The model under review builds one solid part; all positions refer to its coordinate system, in mm. Face numbers are marked on the shaded views. A direction names the side the tool comes from. Coordinates: 2 decimals unless noted, no trailing zeros. Order: outer loops, then holes, each group sorted by start corner. A loop starts at its lowest first (then second) coordinate and runs counter-clockwise, first axis right, second up.
```python
from build123d import *

# Parameters (mm, degrees)
BOSS_EXTRUDE1_DEPTH                      = 42
CBORE_FOR_M64_HEX_HEAD_BOLT1_D           = 70
CBORE_FOR_M64_HEX_HEAD_BOLT1_CBORE_D     = 110
CBORE_FOR_M64_HEX_HEAD_BOLT1_CBORE_DEPTH = 7.5
F_16_5_16_5_DIAMETER_HOLE1_REACH         = 188.325
F_16_5_16_5_DIAMETER_HOLE1_BORE_R        = 8.25
M6_CLEARANCE_HOLE1_D                     = 6.647
M6_CLEARANCE_HOLE1_DEPTH                 = 22.2
M6_CLEARANCE_HOLE1_TIP                   = 1.996960267
CHAMFER1_SIZE                            = 0.5
CHAMFER2_SIZE                            = 1.1765
CHAMFER3_SIZE                            = 0.25


with BuildPart() as part:
    # Sketch1 → Boss-Extrude1 (new body)
    with BuildSketch(Plane(origin=(0, 0, -111.250000238), x_dir=(-1, 0, 0), z_dir=(0, 0, -1))):
        with BuildLine():
            Line((-55.395346272, -72.559925727), (37.878444259, -72.559925727))
            ThreePointArc((37.878444259, -72.559925727), (47.810091488, -64.128468222), (56.241548993, -54.196820993))
            Line((56.241548993, -54.196820993), (56.241548993, 39.076969538))
            ThreePointArc((56.241548993, 39.076969538), (47.810091488, 49.008616768), (37.878444259, 57.440074273))
            Line((37.878444259, 57.440074273), (-55.395346272, 57.440074273))
            ThreePointArc((-55.395346272, 57.440074273), (-65.326993501, 49.008616768), (-73.758451007, 39.076969538))
            Line((-73.758451007, 39.076969538), (-73.758451007, -54.196820993))
            ThreePointArc((-73.758451007, -54.196820993), (-65.326993501, -64.128468222), (-55.395346272, -72.559925727))
        make_face()
    extrude(amount=-BOSS_EXTRUDE1_DEPTH)

    # CBORE for M64 Hex Head Bolt1 (through all)
    with Locations(Plane(origin=(0, 0, -111.250000238), x_dir=(-1, 0, 0), z_dir=(0, 0, -1))):
        with Locations((-8.758451007, -7.559925727)):
            CounterBoreHole(CBORE_FOR_M64_HEX_HEAD_BOLT1_D / 2, CBORE_FOR_M64_HEX_HEAD_BOLT1_CBORE_D / 2, CBORE_FOR_M64_HEX_HEAD_BOLT1_CBORE_DEPTH)

    # Ø16.5 (16.5) Diameter Hole1 bore → Ø16.5 (16.5) Diameter Hole1 (cut, up to next)
    with BuildSketch(Plane(origin=(0, 57.440074273, 0), x_dir=(1, 0, 0), z_dir=(0, 1, 0)), mode=Mode.PRIVATE) as f_16_5_16_5_diameter_hole1_sk1:
        with Locations((-10.241548993, 83.250000238)):
            Circle(F_16_5_16_5_DIAMETER_HOLE1_BORE_R)
    f_16_5_16_5_diameter_hole1_tool1 = extrude(f_16_5_16_5_diameter_hole1_sk1.sketch, amount=-F_16_5_16_5_DIAMETER_HOLE1_REACH, mode=Mode.PRIVATE) & part.part
    add(f_16_5_16_5_diameter_hole1_tool1.solids().sort_by_distance((-10.241549, 57.440074, -83.25))[0], mode=Mode.SUBTRACT)

    # M6 Clearance Hole1
    with Locations(Plane(origin=(0, 0, -111.250000238), x_dir=(-1, 0, 0), z_dir=(0, 0, -1))):
        with Locations((42.506790629, -58.825167363), (-60.023692643, -58.825167363), (-60.023692643, 43.705315909), (42.506790629, 43.705315909)):
            Hole(M6_CLEARANCE_HOLE1_D / 2, depth=M6_CLEARANCE_HOLE1_DEPTH)
            with Locations((0, 0, -(M6_CLEARANCE_HOLE1_DEPTH + M6_CLEARANCE_HOLE1_TIP / 2))):  # 118° drill point
                Cone(0, M6_CLEARANCE_HOLE1_D / 2, M6_CLEARANCE_HOLE1_TIP, mode=Mode.SUBTRACT)

    # Chamfer1
    chamfer1_edges = [part.edges().sort_by_distance(p)[0] for p in [
        (-56.241548993, -7.559925727, -111.250000238),
        (-47.810091488, -64.128468222, -111.250000238),
        (8.758451007, -72.559925727, -111.250000238),
        (65.326993501, -64.128468222, -111.250000238),
        (63.758451007, -7.559925727, -111.250000238),
        (-26.241548993, -7.559925727, -103.750000238),
        (73.758451007, -7.559925727, -111.250000238),
        (65.326993501, 49.008616768, -111.250000238),
        (8.758451007, 57.440074273, -111.250000238),
        (-47.810091488, 49.008616768, -111.250000238),
    ]]
    chamfer(chamfer1_edges, length=CHAMFER1_SIZE)

    # Chamfer2
    chamfer2_edges = [part.edges().sort_by_distance(p)[0] for p in [
        (-45.830290629, 43.705315909, -111.250000238),
        (56.700192643, 43.705315909, -111.250000238),
        (56.700192643, -58.825167363, -111.250000238),
        (-45.830290629, -58.825167363, -111.250000238),
    ]]
    chamfer(chamfer2_edges, length=CHAMFER2_SIZE)

    # Chamfer3
    chamfer3_edges = [part.edges().sort_by_distance(p)[0] for p in [
        (-18.491548993, 57.440074273, -83.250000238),
    ]]
    chamfer(chamfer3_edges, length=CHAMFER3_SIZE)


solid = part.part
```
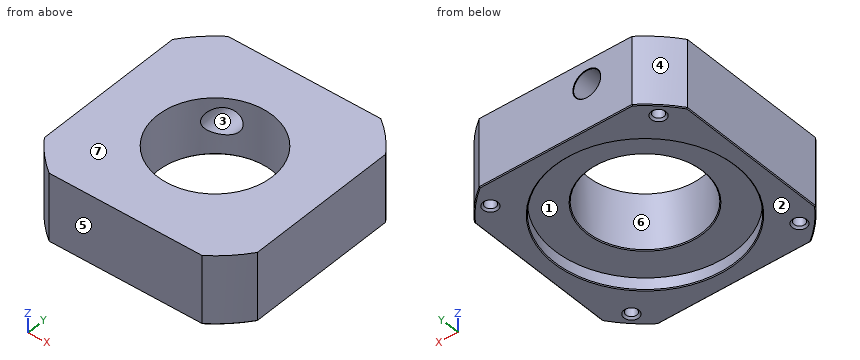
(1) Machinability: for the marked faces 1, 2 and 3, which of the approach directions +Z, -Z, +X, -X, +Y, -Y give a long, thin tool a straight path to every point of the face, cutting with its end or side? Answer none if there is none.
A:
face 1: -Z
face 2: -Z, +X, -X, +Y, -Y
face 3: +Y
(2) We need section C-C, the plane x = -15. Count the separate pieces of the cut face and the enclosed holes in it, and give its area (3 significant figures).
A:
separate pieces: 3
enclosed holes: 0
area: 2,410 mm2
(3) We need section B-B, the plane z = -83.25. Write out the cut boundary in (x, y), and give its area (3 significant figures).
A:
outline: (-56.24, -54.2) arc R80 ccw to (-37.88, -72.56) - (55.4, -72.56) arc R80 ccw to (73.76, -54.2) - (73.76, 39.08) arc R80 ccw to (55.4, 57.44) - (-1.74, 57.44) - (-1.99, 57.19) - (-1.99, 25.75) arc R35 cw (long way) to (-18.49, 14.4) - (-18.49, 57.19) - (-18.74, 57.44) - (-37.88, 57.44) arc R80 ccw to (-56.24, 39.08) - close
area: 11,900 mm2
(4) We need section A-A, the plane z = -73. Write out the cut boundary in (x, y).
A:
outline: (-56.24, -54.2) arc R80 ccw to (-37.88, -72.56) - (55.4, -72.56) arc R80 ccw to (73.76, -54.2) - (73.76, 39.08) arc R80 ccw to (55.4, 57.44) - (-37.88, 57.44) arc R80 ccw to (-56.24, 39.08) - close; hole circle Ø70 at (8.76, -7.56)
(5) For pin 1 Ø6 at (x, y) = (60.02, 43.71) entering from -Z; pin 2 Ø1 at (x, z) = (59.5, -92) entering from -Y; pin 3 Ø15 at (x, z) = (-10.24, -83.25) entering from +Y, all flat-tipped, find the tip position at first contact; note any pin that passes through.
A:
pin 1: stops at z = -88.86
pin 2: stops at y = -69.82
pin 3: stops at y = -30.43
(6) Draft analysis for pull direction Y (two halves, no side actions). For the marked faces 4, 5, 6 and 7, state which applies: released by +Y, released by -Y, zero draft, split by the parting line, or undercut.
A:
face 4: released by +Y
face 5: released by -Y
face 6: undercut
face 7: zero draft
(7) Wall thickness on probe 1 along Y at (x, z) = (7.5, -107); probe 2 along Y at (x, z) = (-40.5, -105); probe 3 along Z at (x, y) = (-27.5, 19.5): over which ranges is each line inside the solid? List them lowest first.
A:
probe 1: y = -72.56 to -62.55, 47.43 to 57.44
probe 2: y = -70.6 to -61.47, -56.18 to -32.03, 16.91 to 41.06, 46.35 to 55.48
probe 3: z = -103.75 to -69.25
